Geometry check sheet. Reference: the model listing, model coordinates, mm. A direction names the side the tool comes from. Coordinates: 2 decimals unless noted, no trailing zeros. Order: outer loops, then holes, each group sorted by start corner. A loop starts at its lowest first (then second) coordinate and runs counter-clockwise, first axis right, second up. Notation, with made-up numbers: (60, 43) - (84, 43) arc R12 ccw to (84, 66) - close; hole circle Ø1 at (23.25, 81.25). An arc over 180 degrees is marked (long way). Put each result on its own line as item: value.
from build123d import *

# Parameters (mm, degrees)
EXTRUDE_1_DEPTH     = 40
CUT_EXTRUDE_START   = -3
CUT_EXTRUDE_1_DEPTH = 24
CUT_EXTRUDE_2_DEPTH = 53.224395281
CUT_EXTRUDE_3_DEPTH = 4
CUT_EXTRUDE_START_2 = 2
CUT_EXTRUDE_6_DEPTH = 50.413883947
CHAMFER_1_SIZE      = 1
FILLET_1_R          = 0.3


# Read off the part's stored shape, not the designer's step: Вырез-Вытянуть1, Отверстие с зазором M31
with BuildPart() as part:
    # Эскиз1 → Бобышка-Вытянуть1 (new body)
    with BuildSketch(Plane.XY):
        Polygon((0, 0), (0, 35), (3, 35), (3, -3), (-21, -3), (-21, 0), align=None)
    extrude(amount=EXTRUDE_1_DEPTH)

    # Вырез-Вытянуть1 outline → Вырез-Вытянуть1 (cut)
    with BuildSketch(Plane.ZY.offset(CUT_EXTRUDE_START)):
        with BuildLine():
            ThreePointArc((29.039844892, 17.152543264), (28.161165235, 15.03122292), (29.039844892, 12.909902577))
            Line((29.039844892, 12.909902577), (40, 1.949747468))
            Line((40, 1.949747468), (40, 35))
            Line((40, 35), (0, 35))
            Line((0, 35), (0, -3))
            Line((0, -3), (9.594408409, -3))
            Line((9.594408409, -3), (3.584000769, 3.01040764))
            Line((3.584000769, 3.01040764), (26.918524548, 26.344931419))
            Line((26.918524548, 26.344931419), (32.575378798, 20.68807717))
            Line((32.575378798, 20.68807717), (29.039844892, 17.152543264))
        make_face()
    extrude(amount=CUT_EXTRUDE_1_DEPTH, mode=Mode.SUBTRACT)

    # Эскиз3 → Вырез-Вытянуть2 (cut, through all)
    with BuildSketch(Plane(origin=(0, -0.286796564, 0.286796564), x_dir=(1, 0, 0), z_dir=(0, 0.7071067811865488, -0.7071067811865462))):
        Polygon((-118.62691727, -47.645487261), (-21, -12.112195311), (-0.533369199, -4.662950904), (97.093548071, 30.870341046), (26.026964172, 226.124175586), (-189.693501169, 147.608347279), align=None)
    extrude(amount=-CUT_EXTRUDE_2_DEPTH, mode=Mode.SUBTRACT)

    # Эскиз4 → Вырез-Вытянуть3 (cut)
    with BuildSketch(Plane(origin=(3, 0, 0), x_dir=(0, 0, -1), z_dir=(1, 0, 0))):
        with BuildLine():
            Line((-28, -3), (-28, -0.192388155))
            Line((-28, -0.192388155), (-22.197084645, 5.610527199))
            ThreePointArc((-22.197084645, 5.610527199), (-20.451501777, 6.899494937), (-20.908116908, 9.02081528))
            Line((-20.908116908, 9.02081528), (-23.736544033, 11.849242405))
            ThreePointArc((-23.736544033, 11.849242405), (-25.857864376, 12.305857536), (-27.146832114, 10.560274668))
            Line((-27.146832114, 10.560274668), (-35.414213562, 2.292893219))
            ThreePointArc((-35.414213562, 2.292893219), (-35.847759065, 1.644046521), (-36, 0.878679656))
            Line((-36, 0.878679656), (-36, -3))
            Line((-36, -3), (-28, -3))
        make_face()
    extrude(amount=-CUT_EXTRUDE_3_DEPTH, mode=Mode.SUBTRACT)

    # Эскиз5 → Вырез-Вытянуть6 (cut, through all)
    with BuildSketch(Plane(origin=(0, -5.943650814, 5.943650814), x_dir=(1, 0, 0), z_dir=(0, -0.7071067811865488, 0.7071067811865464)).offset(CUT_EXTRUDE_START_2)):
        Polygon((0, 30.009937166), (3, 28.918026463), (3, 37.662950904), (0, 37.662950904), align=None)
    extrude(amount=CUT_EXTRUDE_6_DEPTH, mode=Mode.SUBTRACT)

    # Фаска1
    chamfer_1_edges = [part.edges().sort_by_distance(p)[0] for p in [
        (-9, -3, 40),
    ]]
    chamfer(chamfer_1_edges, length=CHAMFER_1_SIZE)

    # Отверстие с зазором M31 outline → Отверстие с зазором M31 (revolve, cut)
    with BuildSketch(Plane(origin=(0, 3.108402615, 9.098433688), x_dir=(0, 1, 0), z_dir=(0, 0, -1))):
        Polygon((0, 0), (1.725, 0), (1.6, 0.125), (1.6, 3), (0, 3), align=None)
    revolve(axis=Axis((0, 3.108402615, 9.098433688), (1, 0, 0)), mode=Mode.SUBTRACT)

    # Hole Wizard M31 2 outline → Hole Wizard M31 2 (revolve, cut)
    with BuildSketch(Plane(origin=(0, 21.493178926, 27.483209999), x_dir=(0, 1, 0), z_dir=(0, 0, -1))):
        Polygon((0, 0), (1.725, 0), (1.6, 0.125), (1.6, 3), (0, 3), align=None)
    revolve(axis=Axis((0, 21.493178926, 27.483209999), (1, 0, 0)), mode=Mode.SUBTRACT)

    # Скругление1
    fillet_1_edges = [part.edges().sort_by_distance(p)[0] for p in [
        (0, 0, 38),
        (0, 0, 17.201010127),
    ]]
    fillet(fillet_1_edges, radius=FILLET_1_R)


solid = part.part
Q1. Depth check by flat-ended pin: pin 1 Ø5 at (y, z) = (3.11, 9.1) entering from -X; pin 2 Ø6 at (x, z) = (-6, 15.5) entering from +Y; pin 3 Ø2.5 at (y, z) = (-1.5, 31) entering from +X. Enter the tip coordinate at first touch or a pass-through.
Answer block:
pin 1: stops at x = 0
pin 2: stops at y = 0
pin 3: stops at x = -1
Q2. Access from +Z, -Z, +X, -X, +Y, -Y to the whole of each face (thin tool, end or side, straight path). Record for faces 4 (the flat face through (-11, 0, 27)), 5 (the flat face through (2, 7.34, 34.07)), 6 (the flat face through (1.521, 10.415, 22.303)), 7 (the cylindrical face through (1.521, 1.654, 35.844)), 8 (the flat face through (1, -1, 36)).
Answer block:
face 4: +Z, -Z, -X, +Y
face 5: +Z, +X
face 6: +X, -X
face 7: +X, -X, -Y
face 8: +X, -Y
Q3. Section check A-A on z = 30. Record the boundary of the cut face in (x, y).
Answer block:
outline: (-21, -3) - (-1, -3) - (-1, 0) - (-21, 0) - close; (0, 7.71) - (3, 7.71) - (3, 10.9) - (0.95, 11.95) - (0, 11.95) - close; (0, 18.11) - (3, 18.11) - (3, 23.26) - (0, 23.26) - close
Q4. Thickness scan on L1, parallel to Y at x = 1.5, z = 13; L2, parallel to Y at x = -15.75, z = 28; L3, parallel to X at y = 15, z = 27. Record the ranges inside material, lowest first. Write a range as [from, to].
Answer block:
L1: y = [-3, 12.43]
L2: y = [-3, 0]
L3: x = [0, 3]
Q5. Section check D-D on x = -15.5. Record the boundary of the cut face in (y, z), then the cut area to 3 significant figures.
Answer block:
outline: (-3, 17.3) - (0, 14.3) - (0, 40) - (-2, 40) - (-3, 39) - close
area: 72.1 mm^2
Q6. Section check C-C on z = 37. Record the boundary of the cut face in (x, y).
Answer block:
outline: (-21, -3) - (3, -3) - (3, 3.9) - (0.95, 4.95) - (0, 4.95) - (0, 0.3) arc R0.3 cw to (-0.3, 0) - (-21, 0) - close
Q7. Section check B-B on z = 21.5. Record the boundary of the cut face in (x, y), then the cut area to 3 significant figures.
Answer block:
outline: (-21, -3) - (3, -3) - (3, 5.78) - (0, 5.78) - (0, 0.3) arc R0.3 cw to (-0.3, 0) - (-21, 0) - close; (0, 9.61) - (3, 9.61) - (3, 20.93) - (0, 20.93) - close
area: 123 mm^2
Q8. Draft check along Z on faces 1 (the flat face through (0.48, 7.51, 34.44)), 2 (the flat face through (1.521, 6.484, 31.223)), 3 (the flat face through (0, 10.2, 21.5)). Enter one of: pulls with the +Z half, pulls with the -Z half, needs draft (parallel to the pull), parting line crosses it, or undercut.
Answer block:
face 1: pulls with the +Z half
face 2: undercut
face 3: needs draft
